Design review of the part shown in the three views and the two pictorial views. Dimensions are in mm from the part's minimum x, y and z. A direction names the side the tool comes from. Coordinates: 2 decimals unless noted, no trailing zeros. Loops run counter-clockwise (first coordinate to the right, second up) from the corner with the lowest first, then second, coordinate; pieces in that order, holes last. Notation, with made-up numbers: (-25.75, -0.75) -> (-6.75, -0.75) arc R23 ccw to (-6.75, 9.25) -> close; hole circle Ø8 at (53, -13). An arc over 180 degrees is marked (long way). One line per item, written item: value. Start each with the question number.
1. Add section D-D on x = 105. Write out the cut boundary in (y, z).
2. Machinability: for the marked faces 1 and 2, which of the approach directions +Z, -Z, +X, -X, +Y, -Y give a long, thin tool a straight path to every point of the face, cutting with its end or side? Answer none if there is none.
3. For probe 1 along Z at (x, y) = (76.5, 105); probe 2 along Y at (x, z) = (64, 10.75); probe 3 along X at (y, z) = (33, 0.5), list the stretches that pass through material, from the lowest coordinate up.
4. Add section C-C on z = 12.25. Write out the cut boundary in (x, y).
5. Add section A-A on x = 57.15. Write out the cut boundary in (y, z), plus the area to 3 significant figures.
6. Insertion check: pin 1 (8 mm diameter, centred on x = 29.5, y = 73, fed in from +Z); pin 2 (3 mm diameter, centred on x = 66.5, z = 8.5, fed in from -Y). Each pin has a flat end and moves straight along its axis. Give the tip position at first contact, or say it passes through.
7. Add section B-B on y = 66. Write out the cut boundary in (x, z).
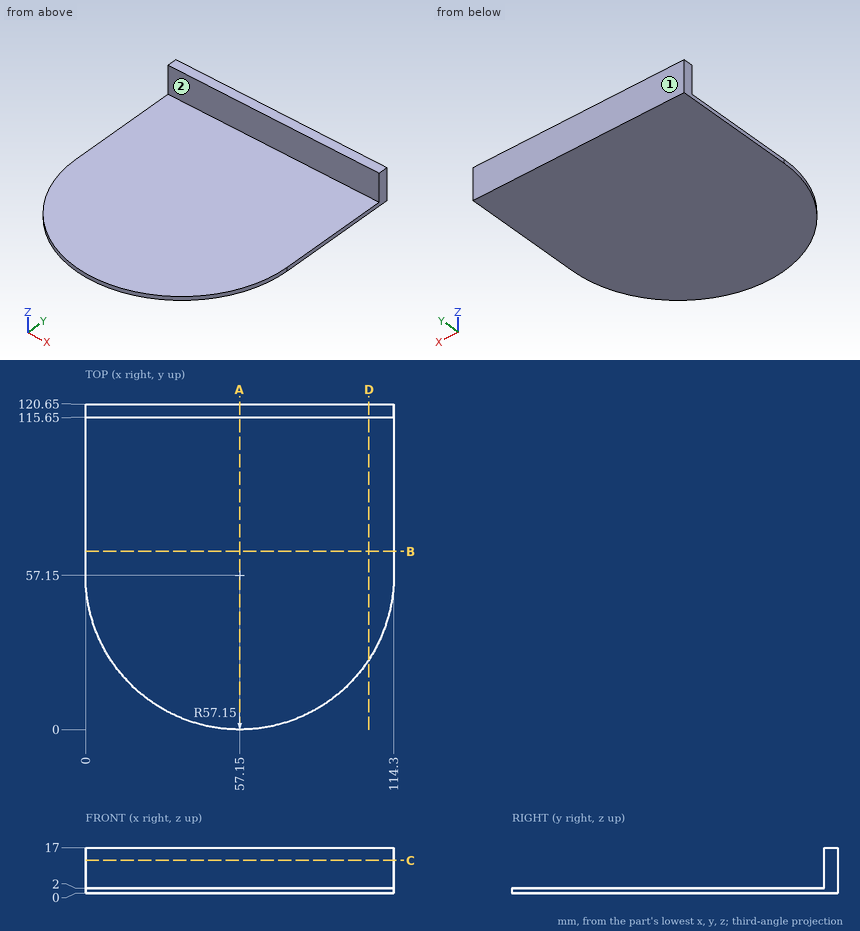
Worked answers:
1. outline: (25.9, 0) -> (120.65, 0) -> (120.65, 17) -> (115.65, 17) -> (115.65, 2) -> (25.9, 2) -> close
2. face 1: +Z, -Z, +X, -X, +Y
2. face 2: +Z, +X, -X, -Y
3. probe 1: z = 0 to 2
3. probe 2: y = 115.65 to 120.65
3. probe 3: x = 5.35 to 108.95
4. outline: (0, 115.65) -> (114.3, 115.65) -> (114.3, 120.65) -> (0, 120.65) -> close
5. outline: (0, 0) -> (120.65, 0) -> (120.65, 17) -> (115.65, 17) -> (115.65, 2) -> (0, 2) -> close
5. area: 316 mm²
6. pin 1: stops at z = 2
6. pin 2: stops at y = 115.65
7. outline: (0, 0) -> (114.3, 0) -> (114.3, 2) -> (0, 2) -> close
